Read the model definition and answer for the solid it produces. Units are mm, in the model's axes. Coordinates: 2 decimals unless noted, no trailing zeros. Order: outer loops, then holes, each group sorted by start corner. A loop starts at its lowest first (then second) coordinate and runs counter-clockwise, first axis right, second up.
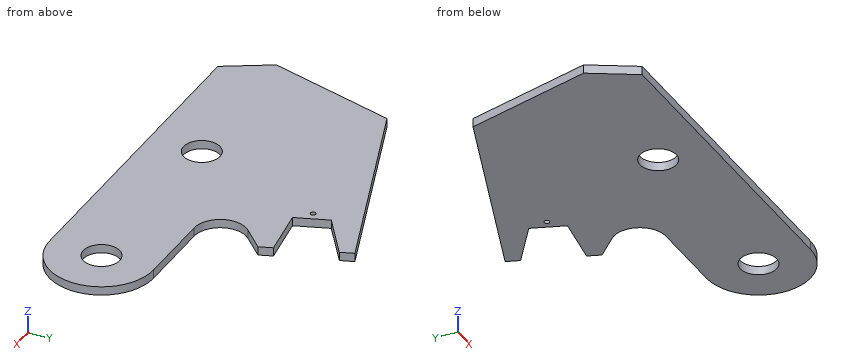
from build123d import *

# Parameters (mm, degrees)
SKETCH1_R           = 10.5
BOSS_EXTRUDE1_DEPTH = 5
FILLET1_R           = 15
SKETCH2_R           = 1.5
CUT_EXTRUDE1_DEPTH  = 5


with BuildPart() as part:
    # Sketch1 → Boss-Extrude1 (new body)
    with BuildSketch(Plane.XY):
        with BuildLine():
            Line((94.301272012, 107.23010703), (12.917479745, 107.23010703))
            Line((12.917479745, 107.23010703), (50.196394157, 144.509021441))
            Line((50.196394157, 144.509021441), (33.09538699, 191.493652481))
            Line((33.09538699, 191.493652481), (-89.064653712, 147.031033848))
            Line((-89.064653712, 147.031033848), (-108.84470723, 73.210869143))
            Line((-108.84470723, 73.210869143), (-93.84470723, 47.23010703))
            Line((-93.84470723, 47.23010703), (94.301272012, 47.23010703))
            ThreePointArc((94.301272012, 47.23010703), (124.301272012, 77.23010703), (94.301272012, 107.23010703))
        make_face()
        with Locations((-17.698727988, 77.23010703)):
            Circle(SKETCH1_R, mode=Mode.SUBTRACT)
        with Locations((94.301272012, 77.23010703)):
            Circle(SKETCH1_R, mode=Mode.SUBTRACT)
    extrude(amount=BOSS_EXTRUDE1_DEPTH)

    # Fillet1
    fillet1_edges = [part.edges().sort_by_distance(p)[0] for p in [
        (12.917479745, 107.23010703, 2.5),
    ]]
    fillet(fillet1_edges, radius=FILLET1_R)

    # Sketch2 → Cut-Extrude1 (cut)
    with BuildSketch(Plane.XY.offset(5)):
        with Locations((9.098668989, 155.090939324)):
            Circle(SKETCH2_R)
        Polygon((35.831548137, 183.976111514), (10.37693066, 166.197966248), (17.217333526, 147.404113833), (47.46023301, 152.026562408), align=None)
    extrude(amount=-CUT_EXTRUDE1_DEPTH, mode=Mode.SUBTRACT)


solid = part.part
Q1. The part is cut by section B-B, the plane x = 97. Determine the outline of the cut face in (y, z), then the cut area to 3 significant figures.
Q2. The part is cut by section C-C, the plane z = 2.4. Determine the outline of the cut face in (x, y), then the cut area to 3 significant figures.
Q3. Straight lines are drawn through the part: L1, parallel to Y at x = 95, z = 1.6; L2, parallel to X at y = 86.5, z = 2.3; L3, parallel to X at y = 77.5, z = 2.85. For each, find the intervals that lie inside material, in ascending order.
Q4. The part is cut by section A-A, the plane y = 84.5. Determine the outline of the cut face in (x, z).
Q5. Each of these flat-tipped pins is pushed along its axis until it touches: P1, Ø2, axis at y = 143.5, z = 4.5, coming from the -X side; P2, Ø12.5, axis at x = -17.7, y = 77.23, coming from the +Z side. Where does it stop, or does it pass through?
Q6. The part is cut by section D-D, the plane x = 41. Determine the outline of the cut face in (y, z), then the cut area to 3 significant figures.
Computed values:
1. outline: (47.35, 0) - (67.08, 0) - (67.08, 5) - (47.35, 5) - close; (87.38, 0) - (107.11, 0) - (107.11, 5) - (87.38, 5) - close
1. area: 197 mm2
2. outline: (-108.84, 73.21) - (-93.84, 47.23) - (94.3, 47.23) arc R30 ccw to (94.3, 107.23) - (49.13, 107.23) arc R15 cw to (38.52, 132.84) - (50.2, 144.51) - (47.46, 152.03) - (17.22, 147.4) - (10.38, 166.2) - (35.83, 183.98) - (33.1, 191.49) - (-89.06, 147.03) - close; hole circle Ø21 at (-17.7, 77.23); hole circle Ø3 at (9.1, 155.09); hole circle Ø21 at (94.3, 77.23)
2. area: 20,200 mm2
3. L1: y = 47.24 to 66.75, 87.71 to 107.22
3. L2: x = -105.28 to -22.63, -12.77 to 89.37, 99.23 to 122.83
3. L3: x = -107.7 to -28.2, -7.2 to 83.8, 104.8 to 124.3
4. outline: (-105.82, 0) - (-25.27, 0) - (-25.27, 5) - (-105.82, 5) - close; (-10.12, 0) - (86.73, 0) - (86.73, 5) - (-10.12, 5) - close; (101.88, 0) - (123.41, 0) - (123.41, 5) - (101.88, 5) - close
5. P1: stops at x = -90.28
5. P2: passes through
6. outline: (47.23, 0) - (109.62, 0) - (109.62, 5) - (47.23, 5) - close; (135.31, 0) - (151.04, 0) - (151.04, 5) - (135.31, 5) - close
6. area: 391 mm2
